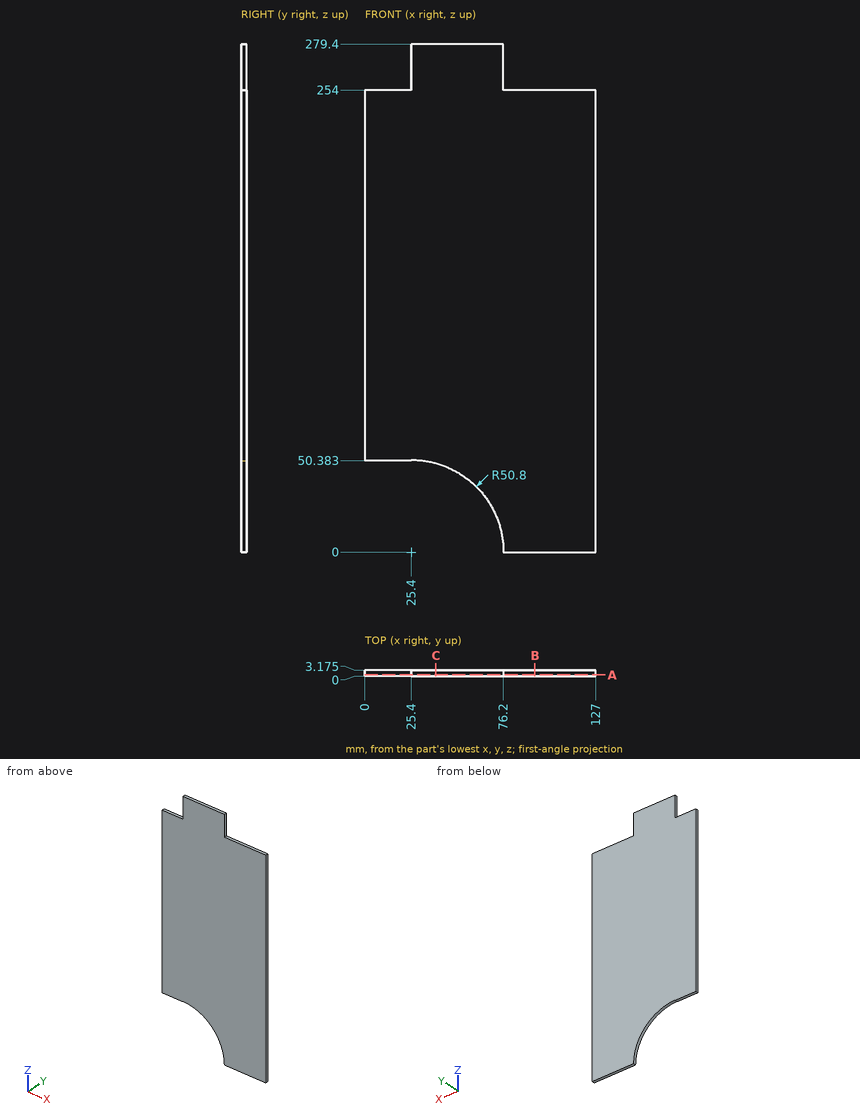
For this review, use the dimensioned drawing (mm, ordinates from the lowest corner) and the shaded views. Coordinates: 2 decimals unless noted, no trailing zeros. Order: outer loops, then holes, each group sorted by start corner. A loop starts at its lowest first (then second) coordinate and runs counter-clockwise, first axis right, second up. Notation, with made-up numbers: M -25,-11.75 L -8,-11.75 A18 ccw -8,11.25 Z; hole C 53.25,7.25 d8. An arc over 180 degrees is marked long. Answer as a JSON object with one key per item and string values. Group by question number.
1) For pin 1 (1 mm diameter, centred on x = 13, y = 1.5, fed in from -Z); pin 2 (1.6 mm diameter, centred on y = 2, z = 267.5, fed in from -X); pin 3 (1.6 mm diameter, centred on y = 1.5, z = 267.5, fed in from +X), all flat-tipped, find the tip position at first contact; note any pin that passes through.
2) Wall thickness on L1, parallel to Z at x = 95, y = 0.7; L2, parallel to X at y = 2.4, z = 263; L3, parallel to Z at x = 47, y = 2.7: over which ranges is each line inside the solid? List them lowest first.
3) Add section A-A, the plane y = 0.55. Write out the cut boundary in (x, z).
4) Add section C-C, the plane x = 39. Write out the cut boundary in (y, z) (1 decimal).
5) Add section B-B, the plane x = 93.5. Write out the cut boundary in (y, z) (1 decimal).
Computed values:
{
 "1": {"pin 1": "stops at z = 50.38", "pin 2": "stops at x = 25.4", "pin 3": "stops at x = 76.2"},
 "2": {"L1": "z = 0 to 254", "L2": "x = 25.4 to 76.2", "L3": "z = 45.98 to 279.4"},
 "3": {"outline": "M 0,50.38 L 25.4,50.38 L 25.4,50.8 A50.8 cw 76.2,0 L 127,0 L 127,254 L 76.2,254 L 76.2,279.4 L 25.4,279.4 L 25.4,254 L 0,254 Z"},
 "4": {"outline": "M 0,48.9 L 3.2,48.9 L 3.2,279.4 L 0,279.4 Z"},
 "5": {"outline": "M 0,0 L 3.2,0 L 3.2,254 L 0,254 Z"}
}
